Here's how the part is built. I have some questions about the finished solid (model axes, mm). A direction names the side the tool comes from. Round coordinates to 2 decimals unless told otherwise and drop trailing zeros. Order: outer loops, then holes, each group sorted by start corner. A loop starts at its lowest first (then second) coordinate and runs counter-clockwise, first axis right, second up. Notation, with made-up numbers: (60.25, -25.5) -> (114.25, -25.5) arc R32 ccw to (114.25, 5.5) -> close; hole circle Ø8 at (-32, 28). An arc over 180 degrees is marked (long way). Use a Markdown table: item, result. Add a question column.
(1) Thinking about a two-plate mould opening in Y: for faces 1 (the face through (-13, 0, 23)), 2 (the face through (-19.139, -25.557, 17.349)), 3 (the face through (-10, -22, 44.45)), which applies, pulls with the +Y half, pulls with the -Y half, needs draft (parallel to the pull), parting line crosses it, or undercut?
(2) I'm going to push flat-ended pins straight in: P1, Ø6, axis at x = -6.5, y = -50.5, coming from the -Z side; P2, Ø4, axis at y = -33, z = 32.5, coming from the -X side; P3, Ø4, axis at x = -20, y = -35.5, coming from the +Z side; P4, Ø3, axis at x = -17.5, z = 31.5, coming from the -Y side. Where does each tip first touch, or does it pass through?
(3) On a 3-axis mill with a long thin cutter (end or side, diameter ignored), from which of +Z, -Z, +X, -X, +Y, -Y can I reach the whole of each face in a straight line? I mean faces 4 (the face through (-19.14, -50.3, 7.99)), 5 (the face through (-13, -28, 0)). Say none if no direction works.
(4) I want a section at A-A, the plane x = -22.5. Please give me the cut outline in (y, z), then the cut area to 3 significant figures.
(5) I want a section at B-B, the plane z = 25.4. Please give me the cut outline in (x, y), then the cut area to 3 significant figures.
(6) If I drill on probe 1 along X at (y, z) = (-44.5, 28); probe 2 along Y at (x, z) = (-22, 25.5); probe 3 along Z at (x, y) = (-14.25, -49.5) (3 decimals), over which ranges is the centre line in solid material (lowest first)?
from build123d import *

# Parameters (mm, degrees)
F0_W     = 25.4
F0_H     = 44.45
F1_DEPTH = 57.15
F3_DEPTH = 12.7
F4_R     = 12.7
F5_DEPTH = 12.7


with BuildPart() as f1:
    # F0 (on Front) → F1 (new body)
    with BuildSketch(Plane.XZ):
        with Locations((-12.7, 22.225)):
            Rectangle(F0_W, F0_H)
    extrude(amount=F1_DEPTH)

    # F2 (on face) → F3 (cut)
    with BuildSketch(Plane(origin=(-25.4, 0, 0), x_dir=(0, -1, 0), z_dir=(-1, 0, 0))):
        Polygon((57.15, 44.45), (19.05, 44.45), (57.15, 0), align=None)
    extrude(amount=-F3_DEPTH, mode=Mode.SUBTRACT)

    # F4 (on face) → F5 (cut)
    with BuildSketch(Plane(origin=(-25.4, 0, 0), x_dir=(0, -1, 0), z_dir=(-1, 0, 0))):
        with Locations((35.378571, 25.4)):
            Circle(F4_R)
    extrude(amount=-F5_DEPTH, mode=Mode.SUBTRACT)


solid = f1.part
Taken from the geometry:
| question | item | result |
|---|---|---|
| 1 | face 1 | pulls with the +Y half |
| 1 | face 2 | undercut |
| 1 | face 3 | needs draft |
| 2 | P1 | stops at z = 0 |
| 2 | P2 | stops at x = -12.7 |
| 2 | P3 | stops at z = 12.88 |
| 2 | P4 | stops at y = -25.2 |
| 3 | face 4 | +Z, -X, -Y |
| 3 | face 5 | -Z, +X, -X, +Y, -Y |
| 4 | outline | (-57.15, 0) -> (0, 0) -> (0, 44.45) -> (-19.05, 44.45) -> (-27.11, 35.04) arc R12.7 cw to (-43.64, 15.76) -> close |
| 4 | area | 1,440 mm2 |
| 5 | outline | (-25.4, -22.68) -> (-12.7, -22.68) -> (-12.7, -57.15) -> (0, -57.15) -> (0, 0) -> (-25.4, 0) -> close |
| 5 | area | 1,010 mm2 |
| 6 | probe 1 | x = -12.7 to 0 |
| 6 | probe 2 | y = -22.68 to 0 |
| 6 | probe 3 | z = 0 to 8.925 |
